Can you work these out from the drawing? Everything is in mm from the part's minimum corner. A direction names the side the tool comes from. Coordinates: 2 decimals unless noted, no trailing zeros. Loops run counter-clockwise (first coordinate to the right, second up) from the corner with the lowest first, then second, coordinate; pieces in that order, holes last. Notation, with made-up numbers: (-32, 87.5) - (-9, 87.5) arc R7 cw to (-9, 98.5) - close; hole circle Ø1 at (-33, -15.5). An arc over 180 degrees is marked (long way). One line per question, with ' | ' between items. Start each with the question number.
1. Which directions (+Z, -Z, +X, -X, +Y, -Y) give clear straight access to the entire face, cutting with the end or side of a thin tool? Please do the marked faces 1, 2 and 3.
2. I want a section at A-A, the plane x = 5.7. Write out the boundary of the cut face in (y, z) (3 decimals).
3. I want a section at C-C, the plane z = 14.25. Write out the boundary of the cut face in (x, y).
4. I want a section at B-B, the plane y = 8.7. Write out the boundary of the cut face in (x, z).
5. Please list where these lines run through material, in increasing order: L1, parallel to Y at x = 8.7, z = 0.65; L2, parallel to Y at x = 8.5, z = 7. Write a range as [from, to].
6. I want a section at D-D, the plane x = 1.75. Write out the boundary of the cut face in (y, z), then the cut area to 3 significant figures.
7. We'd pull the mould along X, two halves only. Please class the marked faces 4, 5 and 6: pulls with the +X half, pulls with the -X half, needs draft (parallel to the pull), parting line crosses it, or undercut.
8. I'm going to push flat-ended pins straight in: P1, Ø5, axis at x = 3.5, z = 13, coming from the -Y side; P2, Ø0.6, axis at x = 10.5, y = 5.5, coming from the +Z side; P3, Ø2, axis at x = 8, z = 3.5, coming from the -Y side. Where does each tip first touch, or does it pass through?
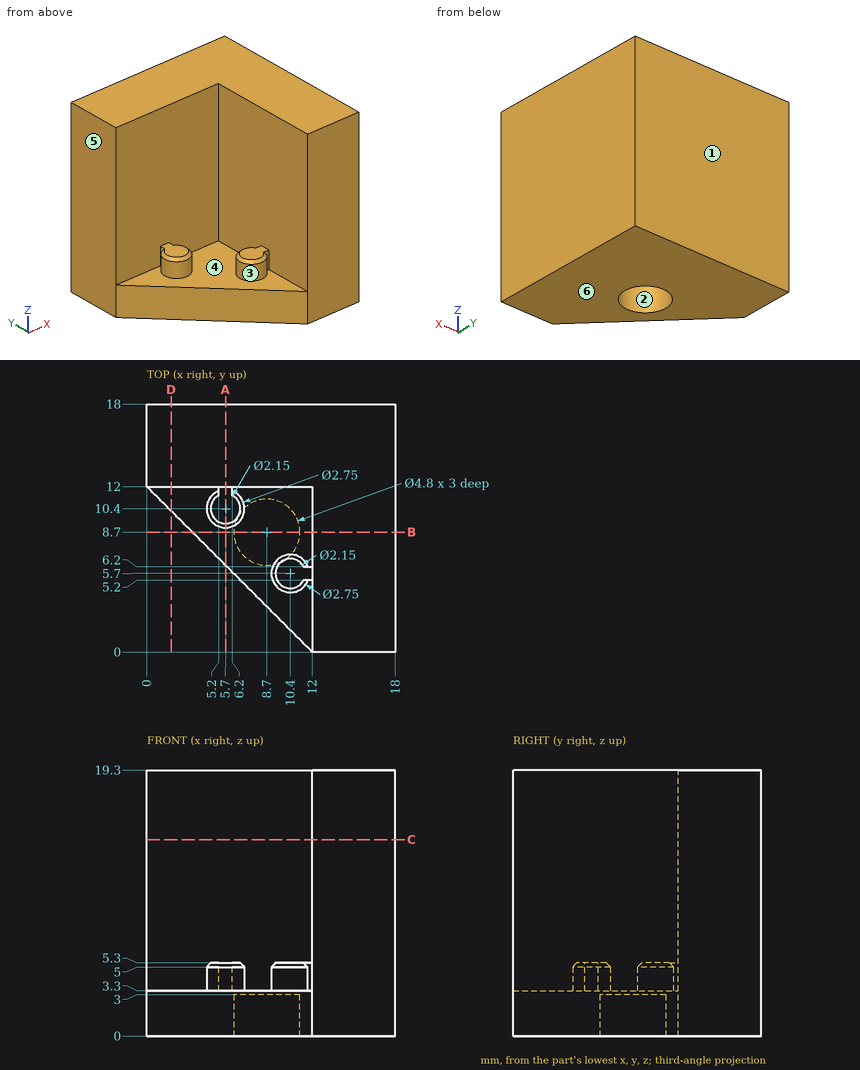
Results are:
1) face 1: +Z, -Z, +X, -X, +Y | face 2: -Z | face 3: +Z
2) outline: (6.3, 0) - (18, 0) - (18, 19.3) - (12, 19.3) - (12, 5.3) - (9.325, 5.3) - (9.025, 5) - (9.025, 3.3) - (6.3, 3.3) - close
3) outline: (0, 12) - (12, 12) - (12, 0) - (18, 0) - (18, 18) - (0, 18) - close
4) outline: (3.3, 0) - (6.3, 0) - (6.3, 3) - (11.1, 3) - (11.1, 0) - (18, 0) - (18, 19.3) - (12, 19.3) - (12, 3.3) - (3.3, 3.3) - close
5) L1: y = [3.3, 6.3], [11.1, 18] | L2: y = [12, 18]
6) outline: (10.25, 0) - (18, 0) - (18, 19.3) - (12, 19.3) - (12, 3.3) - (10.25, 3.3) - close | area: 122 mm2
7) face 4: undercut | face 5: pulls with the -X half | face 6: needs draft
8) P1: stops at y = 12 | P2: stops at z = 5.3 | P3: stops at y = 3.02
